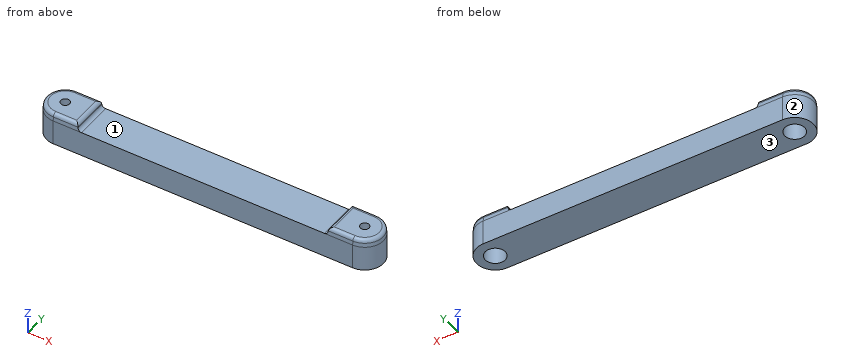
```python
from build123d import *

# Parameters (mm, degrees)
BOSS_EXTRUDE1_DEPTH  = 10
BOSS_EXTRUDE2_DEPTH  = 3
BOSS_EXTRUDE2_TAPER  = 5
FILLET1_R            = 1.5
SKETCH3_R            = 1.75
CUT_EXTRUDE1_DEPTH   = 70.14839116
SKETCH4_R            = 4
CUT_EXTRUDE2_DEPTH   = 10
FILLET1_OF_MIRROR3_R = 1.5
CHAMFER1_SIZE        = 2


with BuildPart() as part:
    # Sketch1 → Boss-Extrude1 (new body)
    with BuildSketch(Plane.XY):
        with BuildLine():
            Line((-60, 7.5), (60, 7.5))
            ThreePointArc((60, 7.5), (67.5, 0), (60, -7.5))
            Line((60, -7.5), (-60, -7.5))
            ThreePointArc((-60, -7.5), (-67.5, 0), (-60, 7.5))
        make_face()
    extrude(amount=BOSS_EXTRUDE1_DEPTH)

    # Sketch2 → Boss-Extrude2 (add)
    with BuildSketch(Plane.XY.offset(10)):
        with BuildLine():
            Line((-50, -7.5), (-50, 7.5))
            Line((-50, 7.5), (-60, 7.5))
            ThreePointArc((-60, 7.5), (-67.5, 0), (-60, -7.5))
            Line((-60, -7.5), (-50, -7.5))
        make_face()
    boss_extrude2 = extrude(amount=BOSS_EXTRUDE2_DEPTH, taper=BOSS_EXTRUDE2_TAPER)

    # Fillet1
    fillet1_edges = [part.edges().sort_by_distance(p)[0] for p in [
        (-50.262465991, 0, 13),
        (-55.131232995, 7.237534009, 13),
        (-67.237534009, 0, 13),
        (-55.131232995, -7.237534009, 13),
        (-50, 0, 10),
    ]]
    fillet(fillet1_edges, radius=FILLET1_R)

    # Sketch3 → Cut-Extrude1 (cut, through all)
    with BuildSketch(Plane.XY.offset(13)):
        with Locations((-60, 0)):
            Circle(SKETCH3_R)
    cut_extrude1 = extrude(amount=-CUT_EXTRUDE1_DEPTH, mode=Mode.SUBTRACT)

    # Sketch4 → Cut-Extrude2 (cut)
    with BuildSketch(Plane(origin=(0, 0, 0), x_dir=(-1, 0, 0), z_dir=(0, 0, -1))):
        with Locations((60, 0)):
            Circle(SKETCH4_R)
    cut_extrude2 = extrude(amount=-CUT_EXTRUDE2_DEPTH, mode=Mode.SUBTRACT)

    # Mirror3: Boss-Extrude2, Cut-Extrude1, Cut-Extrude2 across plane
    add(boss_extrude2.mirror(Plane(origin=(0, 0, 0), x_dir=(0, 0, 1), z_dir=(1, 0, 0))))
    add(cut_extrude1.mirror(Plane(origin=(0, 0, 0), x_dir=(0, 0, 1), z_dir=(1, 0, 0))), mode=Mode.SUBTRACT)
    add(cut_extrude2.mirror(Plane(origin=(0, 0, 0), x_dir=(0, 0, 1), z_dir=(1, 0, 0))), mode=Mode.SUBTRACT)

    # Fillet1 of Mirror3
    fillet1_of_mirror3_edges = [part.edges().sort_by_distance(p)[0] for p in [
        (50.262465991, 0, 13),
        (55.131232995, 7.237534009, 13),
        (67.237534009, 0, 13),
        (55.131232995, -7.237534009, 13),
        (50, 0, 10),
    ]]
    fillet(fillet1_of_mirror3_edges, radius=FILLET1_OF_MIRROR3_R)

    # Chamfer1
    chamfer1_edges = [part.edges().sort_by_distance(p)[0] for p in [
        (56, 0, 10),
        (-56, 0, 10),
    ]]
    chamfer(chamfer1_edges, length=CHAMFER1_SIZE)


solid = part.part
```
Verification items for the finished model (mm, model axes). Face numbers are marked on the shaded views. Round coordinates to 2 decimals unless told otherwise and drop trailing zeros. Write each loop counter-clockwise with the first axis right and the second up, starting at its lowest first coordinate (ties: lowest second). Pieces come first, ordered by that corner, then holes.
1. Section check B-B on x = 38. Enter the section's corners in (y, z).
2. Section check A-A on z = 6.75. Enter the section's corners in (x, y), plus the area to 3 significant figures.
3. Scan lines: L1, parallel to X at y = -2.25, z = 2.25; L2, parallel to Y at x = 60, z = 11.35; L3, parallel to Y at x = -60, z = 6. Record each from-to range of solid material in increasing order.
4. Draft check along X on the marked faces 1, 2 and 3. Enter one of: +X half, -X half, draft (parallel to the pull), parting line (faces both ways), or undercut.
5. Gauge pin test, flat ends, axial feed: P1, Ø4.5, axis at x = -59, y = 0, coming from the -Z side; P2, Ø3, axis at x = 60.5, y = 0.5, coming from the -Z side; P3, Ø2, axis at x = -37.5, y = 0, coming from the +Z side. Record the tip position at first contact, or that the pin passes through.
Answer:
1. outline: (-7.5, 0) - (7.5, 0) - (7.5, 10) - (-7.5, 10) - close
2. outline: (-60, -7.5) - (60, -7.5) arc R7.5 ccw to (60, 7.5) - (-60, 7.5) arc R7.5 ccw to start; hole circle Ø8 at (-60, 0); hole circle Ø8 at (60, 0)
2. area: 1,880 mm2
3. L1: x = -67.15 to -63.31, -56.69 to 56.69, 63.31 to 67.15
3. L2: y = -7.38 to -1.75, 1.75 to 7.38
3. L3: y = -7.5 to -4, 4 to 7.5
4. face 1: undercut
4. face 2: -X half
4. face 3: draft
5. P1: stops at z = 8.75
5. P2: stops at z = 9.79
5. P3: stops at z = 10
